Could you check a few things on this model? Use its own coordinates, in mm. A direction names the side the tool comes from. Round coordinates to 2 decimals unless told otherwise and drop trailing zeros. Write each loop counter-clockwise with the first axis right and the second up, starting at its lowest first coordinate (ties: lowest second). Pieces come first, ordered by that corner, then holes. Notation, with made-up numbers: (21.5, 62) - (75.5, 62) arc R21 ccw to (75.5, 71) - close; hole circle Ø10 at (34, 37). An arc over 180 degrees is marked (long way). Put each result on its own line as item: value.
from build123d import *

# Parameters (mm, degrees)
SKETCH185_R            = 2.6
EXTRUDE200_DEPTH       = 10
SKETCH184_R            = 22.36068
EXTRUDE199_DEPTH       = 20
CUT127_PLACEMENT_ANGLE = 270


with BuildPart() as extrude200:
    # Sketch185 (on Face9 of Cut126) → Extrude200 (new body)
    with BuildSketch(Plane.XY.offset(5.82)):
        Circle(SKETCH185_R)
    extrude(amount=EXTRUDE200_DEPTH)


with BuildPart() as extrude200_1:
    # Extrude200 placement: moved
    add(extrude200.part.moved(Location((0, 0, -7.5))))


with BuildPart() as extrude199:
    # Sketch184 (on Face7 of Revolve005) → Extrude199 (new body)
    with BuildSketch(Plane.XY.offset(20.92)):
        Circle(SKETCH184_R)
    extrude(amount=EXTRUDE199_DEPTH)


with BuildPart() as extrude199_1:
    # Extrude199 placement: moved
    add(extrude199.part.moved(Location((0, 0, -15.1))))


with BuildPart() as obj1:
    # Sketch183 → Revolve005 (revolve)
    with BuildSketch(Plane.XZ):
        Polygon((0, 0), (33.62, 0), (33.62, 3.355495), (32.6, 3.355495), (32.6, 17.564505), (33.62, 17.564505), (33.62, 20.92), (0, 20.92), align=None)
    revolve(axis=Axis((0, 0, 0), (0, 0, 1)))

    # Cut126: cut Extrude199
    add(extrude199_1.part, mode=Mode.SUBTRACT)

    # Cut127: cut Extrude200
    add(extrude200_1.part, mode=Mode.SUBTRACT)


with BuildPart() as obj1_1:
    # Cut127 placement: moved
    add(obj1.part.moved(Location((69.3, 93, 9.45))).rotate(Axis((69.3, 93, 9.45), (1, 0, 0)), CUT127_PLACEMENT_ANGLE))


solid = obj1_1.part
(1) Imagine slicing it at C-C, the plane y = 94.5. List the corners of the cut face in (x, z) for me, then the cut area to 3 significant figures.
Values found:
outline: circle Ø67.24 at (69.3, 9.45); hole circle Ø5.2 at (69.3, 9.45)
area: 3,530 mm^2
(2) I'm going to push flat-ended pins straight in: pin 1 (8.5 mm diameter, centred on x = 69.3, z = 9.45, fed in from +Y); pin 2 (12 mm diameter, centred on y = 103.5, z = -7, fed in from -X); pin 3 (6 mm diameter, centred on x = 63, y = 108.5, fed in from -Z). Where does each tip first touch, or does it pass through?
Values found:
pin 1: stops at y = 98.82
pin 2: stops at x = 38.42
pin 3: stops at z = -23.92
(3) Please list where these lines run through material, in increasing order: probe 1 along X at (y, z) = (104, 9.45); probe 2 along Z at (x, y) = (69.3, 105.75); probe 3 along Z at (x, y) = (69.3, 96.2). Write a range as from..to.
Values found:
probe 1: x = 36.7..46.94, 91.66..101.9
probe 2: z = -23.15..-12.91, 31.81..42.05
probe 3: z = -24.17..6.85, 12.05..43.07
(4) Imagine slicing it at A-A, the plane z = 9.45. List the corners of the cut face in (x, y) for me.
Values found:
outline: (35.68, 93) - (66.7, 93) - (66.7, 98.82) - (46.94, 98.82) - (46.94, 113.92) - (35.68, 113.92) - (35.68, 110.56) - (36.7, 110.56) - (36.7, 96.36) - (35.68, 96.36) - close; (71.9, 93) - (102.92, 93) - (102.92, 96.36) - (101.9, 96.36) - (101.9, 110.56) - (102.92, 110.56) - (102.92, 113.92) - (91.66, 113.92) - (91.66, 98.82) - (71.9, 98.82) - close
(5) If we mould it in two halves opening along X, with no side actions, what happens to faces 1 (the face through (35.713, 94.701, 7.972)), 2 (the face through (69, 98.82, 14)), 3 (the face through (70, 93, 16)), 4 (the face through (71.78, 95.87, 8.67))? For each: pulls with the +X half, pulls with the -X half, needs draft (parallel to the pull), parting line crosses it, or undercut.
Values found:
face 1: parting line crosses it
face 2: undercut
face 3: needs draft
face 4: undercut
(6) Imagine slicing it at B-B, the plane x = 69.3. List the corners of the cut face in (y, z) for me.
Values found:
outline: (93, -24.17) - (96.36, -24.17) - (96.36, -23.15) - (110.56, -23.15) - (110.56, -24.17) - (113.92, -24.17) - (113.92, -12.91) - (98.82, -12.91) - (98.82, 6.85) - (93, 6.85) - close; (93, 12.05) - (98.82, 12.05) - (98.82, 31.81) - (113.92, 31.81) - (113.92, 43.07) - (110.56, 43.07) - (110.56, 42.05) - (96.36, 42.05) - (96.36, 43.07) - (93, 43.07) - close
(7) For faces 5 (the face through (66.39, 106.26, -12.72)), 6 (the face through (102, 110.565, 7)), 7 (the face through (35.713, 112.266, 7.972)), which set-ups out of +Z, -Z, +X, -X, +Y, -Y let a thin tool reach every point of the face, with its end or its side?
Values found:
face 5: +Y
face 6: none
face 7: +Y, -Y
(8) Imagine slicing it at D-D, the plane x = 56. List the corners of the cut face in (y, z) for me, then the cut area to 3 significant figures.
Values found:
outline: (93, -21.43) - (96.36, -21.43) - (96.36, -20.31) - (110.56, -20.31) - (110.56, -21.43) - (113.92, -21.43) - (113.92, -8.53) - (98.82, -8.53) - (98.82, 27.43) - (113.92, 27.43) - (113.92, 40.33) - (110.56, 40.33) - (110.56, 39.21) - (96.36, 39.21) - (96.36, 40.33) - (93, 40.33) - close
area: 717 mm^2
